from build123d import *


with BuildPart() as f1:
    # F0 (on Front) → F1 (revolve)
    with BuildSketch(Plane.XZ):
        with BuildLine():
            Line((0, 0.254), (0, 0))
            Line((0, 0), (49.911, 0))
            ThreePointArc((49.911, 0), (50.539618, 0.260382), (50.8, 0.889))
            Line((50.8, 0.889), (50.8, 20.352157))
            ThreePointArc((50.8, 20.352157), (51.435, 21.59), (50.8, 22.827843))
            Line((50.8, 22.827843), (50.8, 39.37))
            Line((50.8, 39.37), (50.546, 39.37))
            Line((50.546, 39.37), (50.546, 22.689852))
            ThreePointArc((50.546, 22.689852), (51.181, 21.59), (50.546, 20.490148))
            Line((50.546, 20.490148), (50.546, 0.889))
            ThreePointArc((50.546, 0.889), (50.360013, 0.439987), (49.911, 0.254))
            Line((49.911, 0.254), (0, 0.254))
        make_face()
    revolve(axis=Axis((0, 0, 21.369892), (0, 0, 1)))


solid = f1.part
Read the model definition and answer for the solid it produces. Units are mm, in the model's axes. Round coordinates to 2 decimals unless told otherwise and drop trailing zeros. Write each loop counter-clockwise with the first axis right and the second up, starting at its lowest first coordinate (ties: lowest second). Pieces come first, ordered by that corner, then holes.
Q1. Find section C-C on z = 16.5. Determine the outline of the cut face in (x, y).
Values:
outline: circle Ø101.6 at (0, 0); hole circle Ø101.09 at (0, 0)
Q2. Find section A-A on x = 0. Determine the outline of the cut face in (y, z) (3 decimals), and give its area (3 significant figures).
Values:
outline: (-50.8, 0.889) arc R0.889 ccw to (-49.911, 0) - (49.911, 0) arc R0.889 ccw to (50.8, 0.889) - (50.8, 20.352) arc R1.524 ccw to (50.8, 22.828) - (50.8, 39.37) - (50.546, 39.37) - (50.546, 22.69) arc R1.27 cw to (50.546, 20.49) - (50.546, 0.889) arc R0.635 cw to (49.911, 0.254) - (-49.911, 0.254) arc R0.635 cw to (-50.546, 0.889) - (-50.546, 20.49) arc R1.27 cw to (-50.546, 22.69) - (-50.546, 39.37) - (-50.8, 39.37) - (-50.8, 22.828) arc R1.524 ccw to (-50.8, 20.352) - close
area: 45.7 mm2
Q3. Flat-ended cylindrical pins translate along their axes: P1, Ø5, axis at x = -35.5, y = 11.5, coming from the -Z side; P2, Ø2, axis at x = 37.5, z = 22.5, coming from the -Y side; P3, Ø6, axis at x = 24.5, y = 37, coming from the +Z side; P4, Ø10, axis at y = -6.5, z = 8, coming from the -X side. Find the tip coordinate at first contact, or state that the pin passes through.
Values:
P1: stops at z = 0
P2: stops at y = -36.03
P3: stops at z = 0.25
P4: stops at x = -50.78
Q4. The mould has two halves that part along X. Classify faces 1 (the face through (-11.012, -49.592, 10.757)), 2 (the face through (23.324, -44.843, 10.552)), 3 (the face through (1, 1, 0)): released by +X, released by -X, zero draft, split by the parting line, or undercut.
Values:
face 1: split by the parting line
face 2: undercut
face 3: zero draft
Q5. Straight lines are drawn through the part: line 1 (Y direction, x = 0, z = 7.25); line 2 (Z direction, x = 24.5, y = -35); line 3 (Y direction, x = 32, z = 26). For each, find the intervals that lie inside material, in ascending order.
Values:
line 1: y = -50.8 to -50.55, 50.55 to 50.8
line 2: z = 0 to 0.25
line 3: y = -39.45 to -39.13, 39.13 to 39.45
